Source: CAD feature listing. Evaluate the final solid. Frame: model axes, mm. A direction names the side the tool comes from. Coordinates: 2 decimals unless noted, no trailing zeros. Write each loop counter-clockwise with the first axis right and the second up, starting at its lowest first coordinate (ties: lowest second). Pieces come first, ordered by that corner, then holes. Notation, with made-up numbers: M -18.75,31 L 33.25,31 A17 cw 33.25,63 Z; hole C 24.5,34 d6. An arc over 180 degrees is marked long. Answer as CSV lines item,"result". Start each with the question number.
1. Contact query for flat-ended pins moving along their axis: pin 1 Ø12 at (x, y) = (1404, 174.5) entering from +Z; pin 2 Ø3 at (x, z) = (459.5, -54) entering from -Y; pin 3 Ø1.5 at (x, z) = (1269.5, -79.5) entering from +Y. Output: stop coordinate, or through.
2. Mould query, pull axis Z, two halves, no side actions, for faces 1 (the face through (-124.97, 24.65, 2.75)), 2 (the face through (1750, 125, 0)), 3 (the face through (1750, -1, -13)). Classes: pulls with the +Z half, pulls with the -Z half, needs draft (parallel to the pull), parting line crosses it, or undercut.
3. Section A-A on z = 0. Return the cut outline in (x, y).
4. Section B-B on y = 125. Return the cut outline in (x, z), plus the area to 3 significant figures.
5. Section C-C on x = 903. Return the cut outline in (y, z).
6. Section D-D on z = 96. Return the cut outline in (x, y), plus the area to 3 significant figures.
7. Reachability of faces 4 (the face through (45, 50, 2)), 5 (the face through (799, 0, -2)), 6 (the face through (863, 123, 125)), 7 (the face through (799, 250, -2)) from +Z, -Z, +X, -X, +Y, -Y: full face, straight path, thin tool, end or side. Return the list, or none.
8. Line query: probe 1 along Z at (x, y) = (0, 223.5); probe 2 along X at (y, z) = (216.5, 0); probe 3 along Y at (x, z) = (821, -11). Output: solid intervals per line, ascending. Write a range as [from, to].
Autodesk Fusion 360 part; units mm, degrees
sketch "Sketch2" plane through (0, 0, 0) normal (0, 1, 0) x (1, 0, 0)
  line L0 (0, -50) -> (700, -50)
  arc A0 (700, -50) -> (700, 50) centre (700, 0) ccw
  line L1 (700, 50) -> (0, 50)
  arc A1 (0, 50) -> (0, -50) centre (0, 0) ccw
  line L2 (0, 0) -> (700, 0) construction
  circle A2 centre (0, 0) radius 10
  line L3 (700, -50) -> (700, 50)
  dimension "d2" = 100
  dimension "d3" = 20
extrude "Extrude1" add sketch "Sketch2" along normal blind 100 contours L0 L1 A1 L3
sketch "Sketch3" plane through (0, 0, 50) normal (0, 0, 1) x (-1, 0, 0)
  line L0 (0, 0) -> (-700, 0)
  line L1 (-700, 0) -> (-700, -100)
  line L2 (-700, -100) -> (0, -100)
  line L3 (0, -100) -> (0, 0)
  line L4 (-60, -100) -> (-60, 0)
  line L5 (-60, -80) -> (50, -80)
  line L6 (-60, -20) -> (50, -20)
  line L7 (50, -80) -> (50, -20)
  dimension "d6" = 20
  dimension "d7" = 20
extrude "Extrude2" cut sketch "Sketch3" against normal blind 110 contours L3 L5 L6 L7 | L3 L4 L5 L6
sketch "Sketch4" plane through (700, 0, 0) normal (1, 0, 0) x (0, 1, 0)
  line L0 (0, 50) -> (0, -50)
  line L1 (0, -50) -> (100, -50)
  line L2 (100, -50) -> (100, 50)
  line L3 (100, 50) -> (0, 50)
  circle A0 centre (50, 0) radius 75
  dimension "d10" = 150
extrude "Extrude3" add sketch "Sketch4" along normal blind 20 contours L0 L1 L2 L3 | A0
sketch "Sketch5" plane through (720, 0, 0) normal (1, 0, 0) x (0, 1, 0)
  circle A0 centre (50, 0) radius 75
  circle A1 centre (50, 0) radius 10
  dimension "d13" = 20
extrude "Extrude4" cut sketch "Sketch5" against normal blind 20 contours A1
scale "Scale1" factor 2.5 about (0, 0, 0) bodies 1
Values:
1,pin 1,"z = 125"
1,pin 2,"y = 0"
1,pin 3,"y = 250"
2,face 1,"parting line crosses it"
2,face 2,"undercut"
2,face 3,"needs draft"
3,outline,"M -125,0 L -25,0 L -25,50 L -125,50 Z; M -125,200 L -25,200 L -25,250 L -125,250 Z; M 25,0 L 1750,0 L 1750,-62.5 L 1800,-62.5 L 1800,100 L 1750,100 L 1750,150 L 1800,150 L 1800,312.5 L 1750,312.5 L 1750,250 L 25,250 L 25,200 L 150,200 L 150,50 L 25,50 Z"
4,outline,"M 150,-125 L 1750,-125 L 1750,-187.5 L 1800,-187.5 L 1800,-25 L 1750,-25 L 1750,25 L 1800,25 L 1800,187.5 L 1750,187.5 L 1750,125 L 150,125 Z"
4,area,"416,000 mm²"
5,outline,"M 0,-125 L 250,-125 L 250,125 L 0,125 Z"
6,outline,"M -80.06,0 L 1750,0 L 1750,-36.06 L 1800,-36.06 L 1800,286.06 L 1750,286.06 L 1750,250 L -80.06,250 L -80.06,200 L 150,200 L 150,50 L -80.06,50 Z"
6,area,"439,000 mm²"
7,face 4,"+Z, -Z, -X"
7,face 5,"+Z, -Z, -X, -Y"
7,face 6,"+Z, -X, +Y, -Y"
7,face 7,"+Z, -Z, -X, +Y"
8,probe 1,"[-125, -25], [25, 125]"
8,probe 2,"[-125, -25], [25, 1800]"
8,probe 3,"[0, 250]"
